Part model, mm, in its own coordinate system. A direction names the side the tool comes from. Give positions to 0.01 mm unless a question says otherwise; leave off trailing zeros. Write each loop counter-clockwise with the first axis right and the second up, starting at its lowest first coordinate (ties: lowest second). Pieces come first, ordered by that corner, then holes.
from build123d import *

# Parameters (mm, degrees)
F0_R     = 19.05
F0_R_2   = 21.601346
F1_DEPTH = 38.1
F2_DEPTH = 76.2
F3_W     = 40.27349
F3_H     = 2.54
F4_DEPTH = 38.1


with BuildPart() as f1:
    # F0 (on Top) → F1 (new body)
    with BuildSketch(Plane.XY):
        Circle(F0_R)
        Circle(F0_R_2)
        Circle(F0_R, mode=Mode.SUBTRACT)
    extrude(amount=F1_DEPTH)

    # F0 (on Top) → F2 (cut)
    with BuildSketch(Plane.XY):
        Circle(F0_R)
    extrude(amount=F2_DEPTH, mode=Mode.SUBTRACT)

    # F3 (on face) → F4 (join)
    with BuildSketch(Plane.XY):
        with Locations((-0.148629, -0.063356)):
            Rectangle(F3_W, F3_H)
    extrude(amount=F4_DEPTH)


solid = f1.part
1) Saw through at D-D (x = 0). Write the cut outline in (y, z), and give its area (3 significant figures).
Check result:
outline: (-21.6, 0) - (-19.05, 0) - (-19.05, 38.1) - (-21.6, 38.1) - close; (-1.33, 0) - (1.21, 0) - (1.21, 38.1) - (-1.33, 38.1) - close; (19.05, 0) - (21.6, 0) - (21.6, 38.1) - (19.05, 38.1) - close
area: 291 mm2
2) Saw through at A-A (x = 6.5). Write the cut outline in (y, z), and give its area (3 significant figures).
Check result:
outline: (-20.6, 0) - (-17.91, 0) - (-17.91, 38.1) - (-20.6, 38.1) - close; (-1.33, 0) - (1.21, 0) - (1.21, 38.1) - (-1.33, 38.1) - close; (17.91, 0) - (20.6, 0) - (20.6, 38.1) - (17.91, 38.1) - close
area: 302 mm2
3) Mould opens along X. For faces 1 (the flat face through (-2, 0, 0)), 2 (the cylindrical face through (-0.4, -19.046, 18.783)), 3 (the cylindrical face through (-2.812, 21.418, 18.783)) say: +X half, -X half, draft (parallel to the pull), parting line (faces both ways), or undercut.
Check result:
face 1: draft
face 2: undercut
face 3: parting line
4) 3-axis set-ups, long thin cutter, end or side, ignore diameter. For faces 4 (the flat face through (-2, 0, 38.1)), 5 (the cylindrical face through (0.402, 19.046, 18.783)): which of +Z, -Z, +X, -X, +Y, -Y reach the whole face in a straight line?
Check result:
face 4: +Z, +X, -X, +Y, -Y
face 5: +Z, -Z
5) Flat gauge pins, fed straight in: P1, Ø12, axis at x = -17, z = 17.5, coming from the -Y side; P2, Ø1.5, axis at x = 15, z = 11.5, coming from the -Y side; P3, Ø1.5, axis at y = 9, z = 31.5, coming from the +X side. Where does each tip first touch, or does it go through?
Check result:
P1: stops at y = -18.59
P2: stops at y = -16.23
P3: stops at x = 19.96
6) Saw through at C-C (z = 22). Write the cut outline in (x, y), and give its area (3 significant figures).
Check result:
outline: circle Ø43.2 at (0, 0); hole (-19.01, 1.21) - (19.01, 1.21) arc R19.05 ccw to start; hole (-19, -1.33) arc R19.05 ccw to (19, -1.33) - close
area: 423 mm2
7) Drill centre lines: L1, parallel to Y at x = 0, z = 31; L2, parallel to Y at x = 9.5, z = 8.5; L3, parallel to X at y = -3, z = 20. Where is each one in solid material? Low to high.
Check result:
L1: y = -21.6 to -19.05, -1.33 to 1.21, 19.05 to 21.6
L2: y = -19.4 to -16.51, -1.33 to 1.21, 16.51 to 19.4
L3: x = -21.39 to -18.81, 18.81 to 21.39
8) Saw through at B-B (y = 8). Write the cut outline in (x, z).
Check result:
outline: (-20.07, 0) - (-17.29, 0) - (-17.29, 38.1) - (-20.07, 38.1) - close; (17.29, 0) - (20.07, 0) - (20.07, 38.1) - (17.29, 38.1) - close
